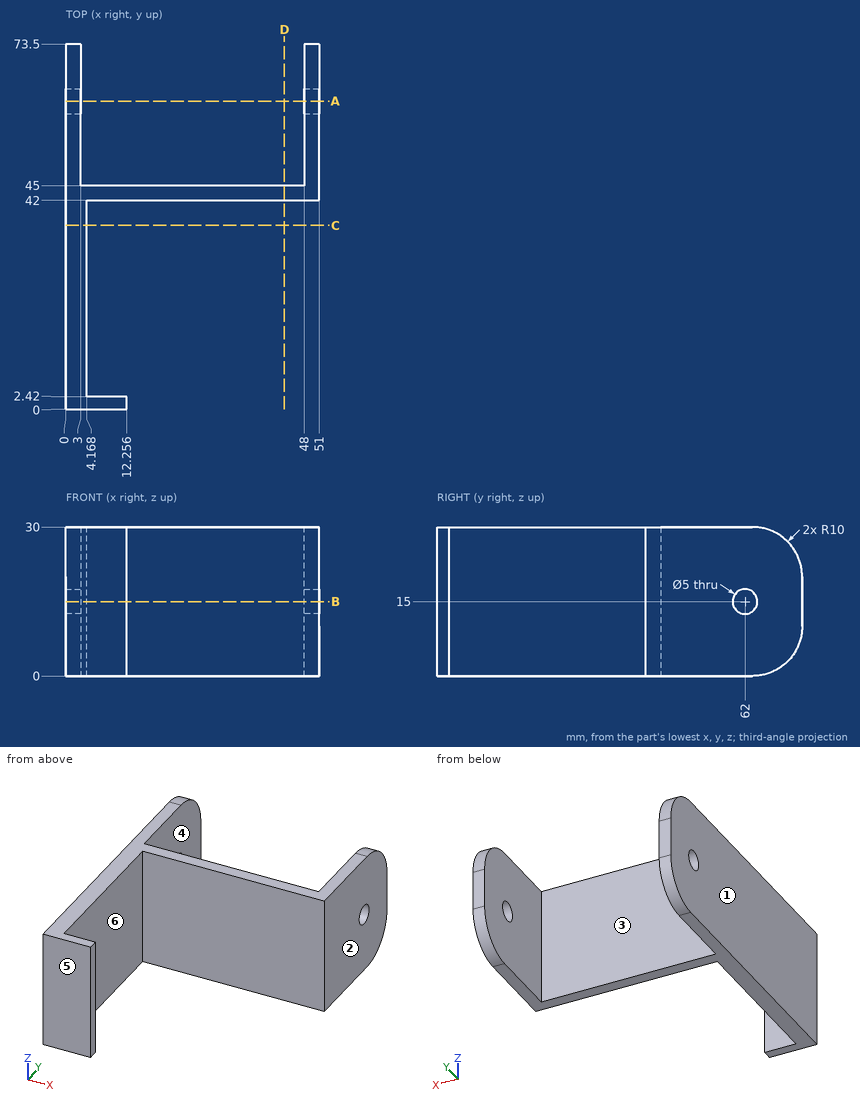
For this review, use the dimensioned drawing (mm, ordinates from the lowest corner) and the shaded views. A direction names the side the tool comes from. Coordinates: 2 decimals unless noted, no trailing zeros. Write each loop counter-clockwise with the first axis right and the second up, starting at its lowest first coordinate (ties: lowest second). Pieces come first, ordered by that corner, then holes. Notation, with made-up numbers: (64, 51) - (117, 51) arc R21 ccw to (117, 76) - close; hole circle Ø9 at (27, -2). An arc over 180 degrees is marked (long way). One line per item, written item: value.
1) Mouldability with a two-part tool opening along X and no side actions: class the marked faces 1, 2 and 3 as +X half, -X half, draft (parallel to the pull), parting line (faces both ways), or undercut.
Answer sheet:
face 1: -X half
face 2: +X half
face 3: undercut
2) Add section D-D (x = 44). State the section outline as (y, z) points.
Answer sheet:
outline: (42, 0) - (45, 0) - (45, 30) - (42, 30) - close
3) Insertion check: pin 1 (6.5 mm diameter, centred on x = 9.5, z = 16.5, fed in from +Y); pin 2 (1.9 mm diameter, centred on y = 1.5, z = 15.5, fed in from +X); pin 3 (6 mm diameter, centred on x = 23.5, z = 19.5, fed in from -Y). Each pin has a flat end and moves straight along its axis. Give the tip position at first contact, or say it passes through.
Answer sheet:
pin 1: stops at y = 45
pin 2: stops at x = 12.26
pin 3: stops at y = 42
4) For the marked faces 4, 5 and 6, list the 3-axis set-ups (+Z, -Z, +X, -X, +Y, -Y) from which the entire face can be reached by the end or side of a thin tool; tool diameter is ignored.
Answer sheet:
face 4: +Z, -Z, +Y
face 5: +Z, -Z, +X, -X, -Y
face 6: +Z, -Z, +X
5) Add section C-C (y = 37). State the section outline as (x, z) points.
Answer sheet:
outline: (0, 0) - (4.17, 0) - (4.17, 30) - (0, 30) - close
6) To check wall thickness, follow probe 1 along X at (y, z) = (50.5, 12.5); probe 2 along Y at (x, z) = (1.15, 15); probe 3 along Y at (x, z) = (4, 26.5). State the ranges of each line that lie inside material, in increasing order.
Answer sheet:
probe 1: x = 0 to 3, 48 to 51
probe 2: y = 0 to 59.5, 64.5 to 73.5
probe 3: y = 0 to 45
7) Add section A-A (y = 62). State the section outline as (x, z) points.
Answer sheet:
outline: (0, 0) - (3, 0) - (3, 12.5) - (0, 12.5) - close; (0, 17.5) - (3, 17.5) - (3, 30) - (0, 30) - close; (48, 0) - (51, 0) - (51, 12.5) - (48, 12.5) - close; (48, 17.5) - (51, 17.5) - (51, 30) - (48, 30) - close
8) Add section B-B (z = 15). State the section outline as (x, y) points.
Answer sheet:
outline: (0, 0) - (12.26, 0) - (12.26, 2.42) - (4.17, 2.42) - (4.17, 42) - (51, 42) - (51, 59.5) - (48, 59.5) - (48, 45) - (3, 45) - (3, 59.5) - (0, 59.5) - close; (0, 64.5) - (3, 64.5) - (3, 73.5) - (0, 73.5) - close; (48, 64.5) - (51, 64.5) - (51, 73.5) - (48, 73.5) - close
